Source: CAD feature listing. Evaluate the final solid. Frame: model axes, mm. A direction names the side the tool comes from. Give positions to 0.01 mm unless a question says otherwise; leave off trailing zeros. Order: outer loops, then holes, each group sorted by start corner. A loop starts at its lowest first (then second) coordinate and runs counter-clockwise, first axis right, second up.
from build123d import *

# Parameters (mm, degrees)
BASEHEAD_DEPTH = 5
BEARINGSKE_W   = 0.8
BEARINGSKE_H   = 8.07179677


with BuildPart() as part:
    # HeadSke → BaseHead (new body)
    with BuildSketch(Plane(origin=(0, 0, 0), x_dir=(0, 0, -1), z_dir=(1, 0, 0))):
        Polygon((6, 3.464101615), (6, -3.464101615), (0, -6.92820323), (-6, -3.464101615), (-6, 3.464101615), (0, 6.92820323), align=None)
    extrude(amount=BASEHEAD_DEPTH)

    # BodySke → BaseBody (revolve)
    with BuildSketch(Plane.XY, mode=Mode.PRIVATE) as basebody_sk:
        Polygon((0, 0), (70, 0), (70, 3), (69, 4), (0, 4), align=None)
    revolve(basebody_sk.sketch.rotate(Axis((0, 0, 0), (1, 0, 0)), 90), axis=Axis((0, 0, 0), (1, 0, 0)))

    # Sketch3 → HeadChamfer (revolve, cut)
    with BuildSketch(Plane(origin=(0, 0, 0), x_dir=(1, 0, 0), z_dir=(0, 1, 0))):
        Polygon((1.5, 8.598076211), (-1.5, 3.401923789), (-13.554766255, 10.361746331), (-10.554766255, 15.557898754), align=None)
    revolve(axis=Axis((0, 0, 0), (1, 0, 0)), mode=Mode.SUBTRACT)

    # BearingSke → BearingFace (revolve, cut)
    with BuildSketch(Plane.XY):
        with Locations((4.6, 10.964101615)):
            Rectangle(BEARINGSKE_W, BEARINGSKE_H)
    revolve(axis=Axis((0, 0, 0), (1, 0, 0)), mode=Mode.SUBTRACT)


solid = part.part
(1) Access query for faces 1 (the cylindrical face through (36.552, 3.905, -0.867)), 2 (the conical face through (0.13, -3.1, 5.4)). Directions: +Z, -Z, +X, -X, +Y, -Y. A direction counts if a zero-diameter tool reaches every point of the face in a straight line with its end or side. Return the directions, or none.
(2) Line query: line 1 along X through (y, z) = (-2, -4); line 2 along Y through (x, z) = (46, -0.25); line 3 along Z through (x, y) = (10.5, 0.75). Output: solid intervals per line, ascending.
(3) Section A-A, the plane x = 32.5. Return loops of the section in (y, z).
(4) Pin query (flat end, axial travel): pin 1 Ø6 at (y, z) = (4.5, -2) entering from -X; pin 2 Ø6 at (x, y) = (26.5, 5.5) entering from -Z; pin 3 Ø8 at (x, y) = (22.5, 2.5) entering from -Z; pin 4 Ø2 at (x, y) = (60, 3) entering from -Z. Return the tip coordinate at first contact, or that it passes through.
Checks:
1. face 1: +X
1. face 2: +Z, -X, -Y
2. line 1: x = 0 to 5
2. line 2: y = -3.99 to 3.99
2. line 3: z = -3.93 to 3.93
3. outline: circle Ø8 at (0, 0)
4. pin 1: stops at x = 0
4. pin 2: stops at z = -3.12
4. pin 3: stops at z = -4
4. pin 4: stops at z = -3.46
